For this review, use the dimensioned drawing (mm, ordinates from the lowest corner) and the shaded views. A direction names the side the tool comes from. Coordinates: 2 decimals unless noted, no trailing zeros. Loops run counter-clockwise (first coordinate to the right, second up) from the corner with the lowest first, then second, coordinate; pieces in that order, holes last. Notation, with made-up numbers: (13, -33.5) -> (72, -33.5) arc R21 cw to (72, -20.5) -> close; hole circle Ø5 at (50.25, 59). An arc over 180 degrees is marked (long way). Answer as a JSON object with one key per item and string values.
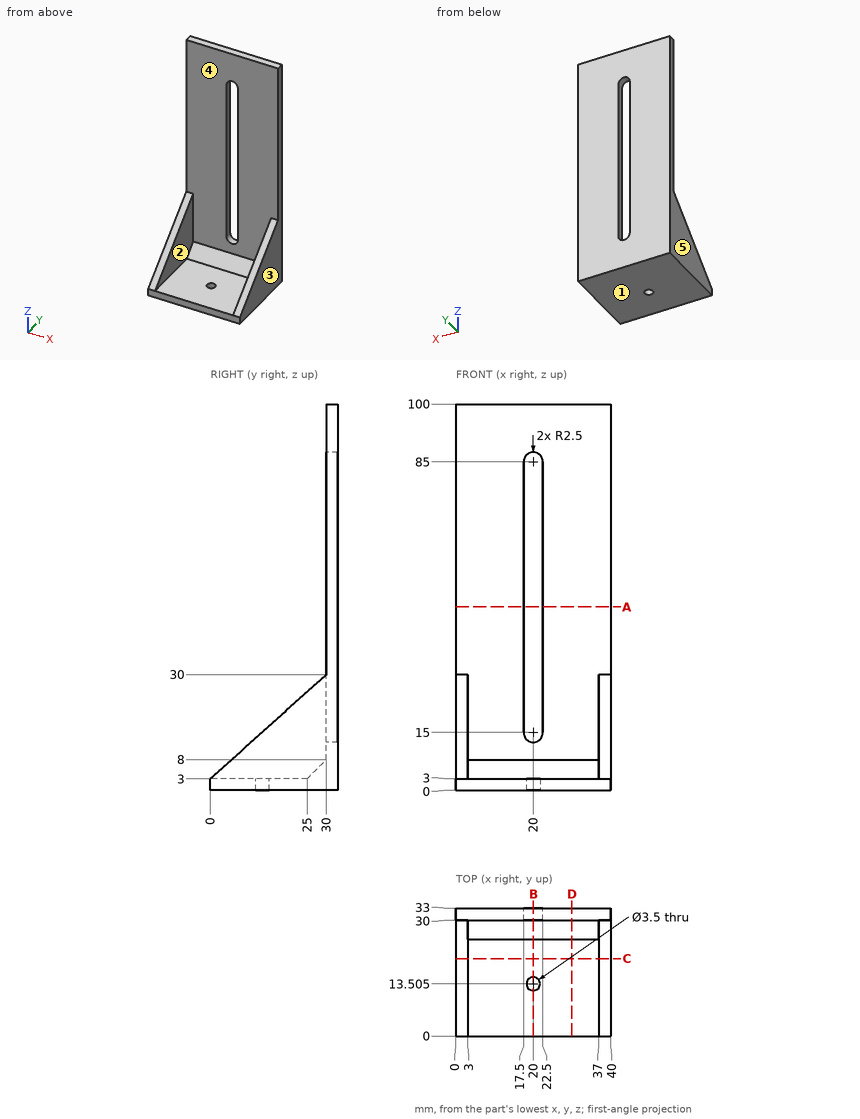
1) Add section B-B, the plane x = 20. Give the boundary of the cut face in (y, z) (1 decimal), and give its area (3 significant figures).
Completed:
{"outline": "(0, 0) -> (11.8, 0) -> (11.8, 3) -> (0, 3) -> close; (15.3, 0) -> (33, 0) -> (33, 12.5) -> (30, 12.5) -> (30, 8) -> (25, 3) -> (15.3, 3) -> close; (30, 87.5) -> (33, 87.5) -> (33, 100) -> (30, 100) -> close", "area": "167 mm²"}
2) Clearance check with a flat-ended pin moving along its axis: pin 1 Ø20 at (x, z) = (29, 37.5) entering from -Y. State where the tip first meets the part, or that it passes through.
Completed:
{"pin 1": "y = 30"}
3) Wall thickness on probe 1 along Y at (x, z) = (20, 2.05) (1 decimal); probe 2 along X at (y, z) = (23.5, 22.5); probe 3 along Y at (x, z) = (6.5, 83.5): over which ranges is each line inside the solid? List them lowest first.
Completed:
{"probe 1": "0 to 11.8, 15.3 to 33", "probe 2": "0 to 3, 37 to 40", "probe 3": "30 to 33"}
4) Add section D-D, the plane x = 30. Give the boundary of the cut face in (y, z).
Completed:
{"outline": "(0, 0) -> (33, 0) -> (33, 100) -> (30, 100) -> (30, 8) -> (25, 3) -> (0, 3) -> close"}
5) Add section A-A, the plane z = 47.5. Give the boundary of the cut face in (x, y), and give its area (3 significant figures).
Completed:
{"outline": "(0, 30) -> (17.5, 30) -> (17.5, 33) -> (0, 33) -> close; (22.5, 30) -> (40, 30) -> (40, 33) -> (22.5, 33) -> close", "area": "105 mm²"}
6) For the marked faces 4 and 5, list the 3-axis set-ups (+Z, -Z, +X, -X, +Y, -Y) from which the entire face can be reached by the end or side of a thin tool; tool diameter is ignored.
Completed:
{"face 4": "+Z, -Y", "face 5": "+Z, -Z, -X, +Y, -Y"}
7) The part is to be moulded in two halves that separate along X. For the marked faces 1, 2 and 3, say which applies: pulls with the +X half, pulls with the -X half, needs draft (parallel to the pull), parting line crosses it, or undercut.
Completed:
{"face 1": "needs draft", "face 2": "undercut", "face 3": "pulls with the +X half"}
8) Add section C-C, the plane y = 20. Give the boundary of the cut face in (x, z), and give its area (3 significant figures).
Completed:
{"outline": "(0, 0) -> (40, 0) -> (40, 21) -> (37, 21) -> (37, 3) -> (3, 3) -> (3, 21) -> (0, 21) -> close", "area": "228 mm²"}
